Geometry: final body of the model. Coordinates: model frame, mm. Face numbers are marked on the shaded views. A direction names the side the tool comes from. Round coordinates to 2 decimals unless told otherwise and drop trailing zeros. Order: outer loops, then holes, each group sorted by start corner. A loop starts at its lowest first (then second) coordinate and runs counter-clockwise, first axis right, second up. Notation, with made-up numbers: M -20,-36 L 6,-36 A11 cw 6,-31 Z; hole C 3,21.25 d11. An arc over 180 degrees is marked long. Put each result on its own line as item: value. Start each with the question number.
1) First-contact query: P1, Ø4, axis at x = 5, y = 5.5, coming from the -Z side; P2, Ø12, axis at x = 6.5, z = -53.5, coming from the -Y side; P3, Ø3.5, axis at x = -0.5, y = 8.5, coming from the +Z side. Flat tips, straight axial feed; report the tip coordinate or a pass-through.
2) Section C-C, the plane y = -9.5. Return loops of the section in (x, z).
3) Section A-A, the plane z = -23.5. Return loops of the section in (x, y), then the cut area to 3 significant figures.
4) Draft query along X for the marked faces 1, 2, 3 and 4. Return one class per face: pulls with the +X half, pulls with the -X half, needs draft (parallel to the pull), parting line crosses it, or undercut.
5) Section B-B, the plane x = -10. Return loops of the section in (y, z).
6) Material intervals for probe 1 along Y at (x, z) = (-14, 0); probe 2 along X at (y, z) = (3.25, -10); probe 3 along X at (y, z) = (7.25, -47.5), sorted ascending. Write a range as [from, to].
7) Access query for the marked faces 5, 6, 7 and 8. Directions: +Z, -Z, +X, -X, +Y, -Y. A direction counts if a zero-diameter tool reaches every point of the face in a straight line with its end or side. Return the directions, or none.
from build123d import *

# Parameters (mm, degrees)
F0_R     = 7.5
F1_DEPTH = 16
F3_W     = 15.3093371987
F3_H     = 50
F4_DEPTH = 55.501
F5_R     = 4
F6_DEPTH = 55.501


# Not quite as in the source:
# - a feature names something its author has since deleted; it is built from what else it names


with BuildPart() as f1:
    # F0 (on Right) → F1 (new body, symmetric)
    with BuildSketch(Plane.YZ):
        with BuildLine():
            Line((15, -85), (15, 0))
            ThreePointArc((15, 0), (-11.6189500386, 9.4868329805), (3, -14.6969384567))
            Line((3, -14.6969384567), (3, -85))
            Line((3, -85), (15, -85))
        make_face()
        Circle(F0_R, mode=Mode.SUBTRACT)
    extrude(amount=F1_DEPTH, both=True)

    # F3 (on offset) → F4 (cut, through all)
    with BuildSketch(Plane.XZ.offset(40.5)):
        with BuildLine():
            Line((6.3565325715, -68.9971852547), (6.3456283358, -44.3721764072))
            Line((6.3456283358, -44.3721764072), (6.3452962394, -43.6222039062))
            ThreePointArc((6.3452962394, -43.6222039062), (-0.1889815849, -37.6462766652), (-6.3565331947, -44))
            Line((-6.3565331947, -44), (-6.3565331947, -69))
            ThreePointArc((-6.3565331947, -69), (0, -75.3565331947), (6.3565331947, -69))
            ThreePointArc((6.3565331947, -69), (6.3565330389, -68.9985926273), (6.3565325715, -68.9971852547))
        make_face()
        Rectangle(F3_W, F3_H)
    extrude(amount=-F4_DEPTH, mode=Mode.SUBTRACT)

    # F5
    f5_edges = [f1.edges().sort_by_distance(p)[0] for p in [
        (-11.827334, 3, -14.696938),
        (11.827334, 3, -14.696938),
    ]]
    fillet(f5_edges, radius=F5_R)

    # F3 (on offset) → F6 (cut, through all)
    with BuildSketch(Plane.XZ.offset(40.5)):
        with BuildLine():
            ThreePointArc((2.313e-07, -85), (-11.3137084172, -80.3137085808), (-16, -69))
            Line((-16, -69), (-16, -85))
            Line((-16, -85), (2.313e-07, -85))
        make_face()
        with BuildLine():
            ThreePointArc((16, -69), (11.3137085808, -80.3137084172), (2.313e-07, -85))
            Line((2.313e-07, -85), (16, -85))
            Line((16, -85), (16, -69))
        make_face()
        with BuildLine():
            Line((6.3565325715, -68.9971852547), (6.3456283358, -44.3721764072))
            Line((6.3456283358, -44.3721764072), (6.3452962394, -43.6222039062))
            ThreePointArc((6.3452962394, -43.6222039062), (-0.1889815849, -37.6462766652), (-6.3565331947, -44))
            Line((-6.3565331947, -44), (-6.3565331947, -69))
            ThreePointArc((-6.3565331947, -69), (0, -75.3565331947), (6.3565331947, -69))
            ThreePointArc((6.3565331947, -69), (6.3565330389, -68.9985926273), (6.3565325715, -68.9971852547))
        make_face()
        Rectangle(F3_W, F3_H)
    extrude(amount=-F6_DEPTH, mode=Mode.SUBTRACT)


solid = f1.part
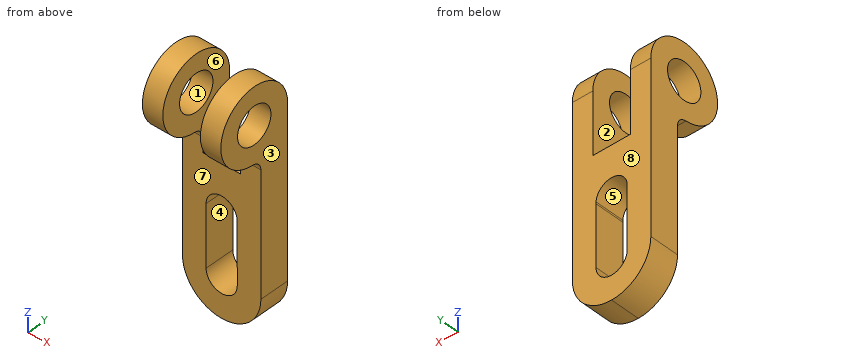
Result sheet:
1. P1: stops at z = -84.72
1. P2: stops at y = 3
1. P3: stops at z = -25
2. outline: M -16,-11.61 L -7.65,-11.61 L -7.65,11.61 L -16,11.61 Z; M 7.65,-11.61 L 16,-11.61 L 16,11.61 L 7.65,11.61 Z
3. outline: M -16,3 L -7.65,3 L -7.65,15 L -16,15 Z; M 7.65,3 L 16,3 L 16,15 L 7.65,15 Z
3. area: 200 mm2
4. face 1: needs draft
4. face 2: undercut
4. face 3: pulls with the +X half
4. face 4: undercut
5. outline: M -0.79,-14.98 A4 cw 3,-18.97 L 3,-81.49 L 15,-81.49 L 15,0 A15 ccw long Z; hole C 0,0 d15
6. probe 1: y = [-15, -7.5], [7.5, 15]
6. probe 2: x = [-16, -7.65], [7.65, 16]
6. probe 3: x = [-16, -6.36], [6.35, 16]
7. face 5: +Y, -Y
7. face 6: +Z, +Y, -Y
7. face 7: -Z, +X, -X, -Y
7. face 8: +Z, -Z, +X, -X, +Y
